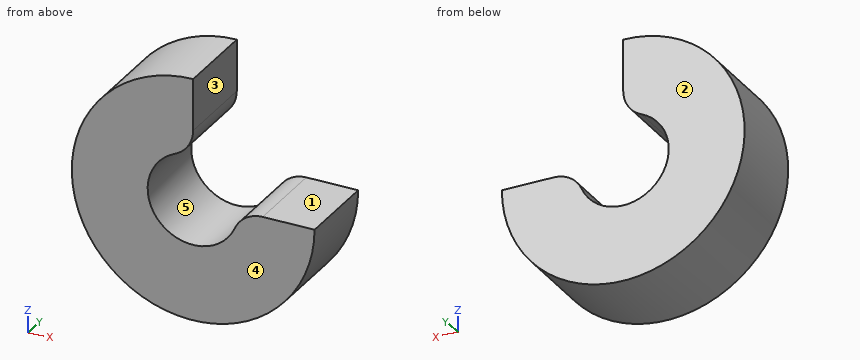
```python
from build123d import *

# Parameters (mm, degrees)
SALIENTE_EXTRUIR1_DEPTH = 2.75
REDONDEO1_R             = 1


with BuildPart() as part:
    # Croquis1 → Saliente-Extruir1 (new body)
    with BuildSketch(Plane(origin=(0, 0, 0), x_dir=(1, 0, 0), z_dir=(0, 1, 0))):
        with BuildLine():
            Line((1.5, 0), (4, 0))
            ThreePointArc((4, 0), (-2.828427125, 2.828427125), (0, -4))
            Line((0, -4), (0, -1.5))
            ThreePointArc((0, -1.5), (-1.060660172, 1.060660172), (1.5, 0))
        make_face()
    extrude(amount=SALIENTE_EXTRUIR1_DEPTH)

    # Redondeo1
    redondeo1_edges = [part.edges().sort_by_distance(p)[0] for p in [
        (0, 1.375, 1.5),
        (1.5, 1.375, 0),
    ]]
    fillet(redondeo1_edges, radius=REDONDEO1_R)


solid = part.part
```
For this review, take the finished solid that the model builds, in its own axes (mm). Face numbers are marked on the shaded views. A direction names the side the tool comes from. Round coordinates to 2 decimals unless told otherwise and drop trailing zeros. Write each loop counter-clockwise with the first axis right and the second up, starting at its lowest first coordinate (ties: lowest second). Pieces come first, ordered by that corner, then holes. Notation, with made-up numbers: (69, 23) - (89, 23) arc R13 ccw to (89, 39) - close; hole circle Ø7 at (68.25, 18). An arc over 180 degrees is marked (long way). Put each result on its own line as item: value.
Q1. Wall thickness on probe 1 along X at (y, z) = (1.9, -1); probe 2 along Z at (x, y) = (-0.5, 2.4); probe 3 along Z at (x, y) = (-0.75, 2.65): over which ranges is each line inside the solid? List them lowest first.
Solved:
probe 1: x = -3.87 to -1.12, 1.12 to 3.87
probe 2: z = -3.97 to -1.41, 1.43 to 3.97
probe 3: z = -3.93 to -1.3, 1.3 to 3.93
Q2. Mouldability with a two-part tool opening along X and no side actions: class the marked faces 3, 4 and 5 as released by +X, released by -X, zero draft, split by the parting line, or undercut.
Solved:
face 3: released by +X
face 4: zero draft
face 5: undercut
Q3. We need section D-D (x = 0.75). Give the boundary of the cut face in (y, z), and give its area (3 significant figures).
Solved:
outline: (0, -3.93) - (2.75, -3.93) - (2.75, -1.3) - (0, -1.3) - close
area: 7.23 mm2
Q4. We need section A-A (z = -0.25). Give the boundary of the cut face in (x, y), and give its area (3 significant figures).
Solved:
outline: (-3.99, 0) - (-1.48, 0) - (-1.48, 2.75) - (-3.99, 2.75) - close; (1.63, 0) - (3.99, 0) - (3.99, 2.75) - (1.63, 2.75) - close
area: 13.4 mm2
Q5. We need section B-B (y = 2.2). Give the boundary of the cut face in (x, z), and give its area (3 significant figures).
Solved:
outline: (-0.6, 1.37) arc R1 ccw to (0, 2.29) - (0, 4) arc R4 ccw (long way) to (4, 0) - (2.29, 0) arc R1 ccw to (1.37, -0.6) arc R1.5 cw (long way) to start
area: 32.2 mm2
Q6. Machinability: for the marked faces 1 and 2, which of the approach directions +Z, -Z, +X, -X, +Y, -Y give a long, thin tool a straight path to every point of the face, cutting with its end or side? Answer none if there is none.
Solved:
face 1: +Z, +X, +Y, -Y
face 2: +Z, -Z, +X, -X, +Y
Q7. Insertion check: pin 1 Ø0.9 at (x, y) = (3, 1.5) entering from +Z; pin 2 Ø2.5 at (x, z) = (0, 0) entering from +Y; pin 3 Ø0.9 at (y, z) = (1.5, 3) entering from +X. Each pin has a flat end and moves straight along its axis. Give the tip position at first contact, or say it passes through.
Solved:
pin 1: stops at z = 0
pin 2: passes through
pin 3: stops at x = 0
Q8. We need section C-C (x = 2). Give the boundary of the cut face in (y, z), and give its area (3 significant figures).
Solved:
outline: (0, -3.46) - (2.75, -3.46) - (2.75, -0.04) - (0, -0.04) - close
area: 9.41 mm2
